Work out the finished part from the listing and answer in its coordinate system (mm). Give positions to 0.01 mm unless a question says otherwise; leave off trailing zeros. Order: outer loops, then holes, each group sorted by start corner. A loop starts at its lowest first (then second) coordinate and runs counter-clockwise, first axis right, second up. Notation, with made-up numbers: (31.25, -28.5) -> (74.25, -28.5) arc R32 cw to (74.25, -0.5) -> close; hole circle Ø5 at (-31, 1). An arc over 180 degrees is marked (long way). Answer as CSV lines item,"result". Start each with the question number.
1. A cutting plane is placed at A-A (z = 1147.5). Give the vertices of the cut face in (x, y), then the cut area to 3 significant figures.
2. A cutting plane is placed at C-C (y = 27). Give the vertices of the cut face in (x, z), then the cut area to 3 significant figures.
3. A cutting plane is placed at B-B (x = 15.5). Give the vertices of the cut face in (y, z).
4. Flat-ended cylindrical pins translate along their axes: pin 1 (3 mm diameter, centred on x = 6.5, y = 11, fed in from +Z); pin 2 (1.5 mm diameter, centred on y = 28, z = 1236.5, fed in from +X); pin 3 (8 mm diameter, centred on x = 25, z = 731, fed in from +Y). Find the tip coordinate at first contact, or state that the pin passes through.
5. Find the intervals of material crossed by L1, parallel to X at y = 3.5, z = 1756; L2, parallel to X at y = 26, z = 1172, in increasing order.
Autodesk Inventor part; units mm, degrees
ref_plane "Start plane" through (0, 0, 0) normal (0, 0, 1) x (1, 0, 0)
ref_plane "End plane" through (0, 0, 1841.5) normal (0, 0, 1) x (1, 0, 0)
ref_plane "Work Plane4" through (19.05, 0, 0) normal (0, 0.7071, -0.7071) x (1, 0, 0)
ref_plane "Start plane" through (0, 0, 0) normal (0, 0, 1) x (1, 0, 0)
ref_plane "End plane" through (0, 0, 1841.5) normal (0, 0, 1) x (1, 0, 0)
sketch "Sketch" plane through (0, 0, 0) normal (0, 0, 1) x (1, 0, 0)
  line L0 (38.1, 0) -> (0, 0)
  line L1 (0, 0) -> (0, 38.1)
  line L2 (0, 38.1) -> (2.4765, 38.1)
  line L3 (4.7625, 35.814) -> (4.7625, 9.5885)
  line L4 (9.5885, 4.7625) -> (35.814, 4.7625)
  line L5 (38.1, 2.4765) -> (38.1, 0)
  line L6 (0, -11.0414) -> (0, 31.5385) construction
  line L7 (-11.0414, 0) -> (31.5385, 0) construction
  arc A0 (4.7625, 9.5885) -> (9.5885, 4.7625) centre (9.5885, 9.5885) ccw
  arc A1 (4.7625, 35.814) -> (2.4765, 38.1) centre (2.4765, 35.814) ccw
  arc A2 (38.1, 2.4765) -> (35.814, 4.7625) centre (35.814, 2.4765) ccw
  line L8 (0, 48.4964) -> (0, -20.9644) construction
  line L9 (-20.9644, 0) -> (48.4964, 0) construction
  point P0 (4.7625, 38.1)
  point P1 (4.7625, 4.7625)
  point P2 (38.1, 4.7625)
  dimension "d0" = 38.1
  dimension "d1" = 38.1
  dimension "d2" = 4.7625
  dimension "d3" = 4.7625
  dimension "d10" = 0
  dimension "d11" = 0
  dimension "d14" = 4.826
  dimension "d15" = 2.286
extrude "Body" add sketch "Sketch" along normal up to surface (1841.5 mm away) from surface at 0
sketch "Sketch3" plane through (0, 0, 0) normal (0, 0, 1) x (1, 0, 0)
  line L0 (0, 0) -> (10, 0)
ref_plane "Work Plane3" through (0, 0, 0) normal (0, -1, 0) x (1, 0, 0)
sketch "Sketch4" plane through (0, 0, 0) normal (0, -1, 0) x (1, 0, 0)
  line L0 (-2, 0) -> (12, 0)
  line L1 (-2, 1841.5) -> (12, 1841.5)
  dimension "d17" = 1841.5
ref_plane "Work Plane4" through (19.05, 0, 0) normal (0, 0.7071, -0.7071) x (1, 0, 0)
split "Split1" plane through (19.05, 0, 0) removes the side toward (0, 0.7071, -0.7071)
ref_plane "Work Plane5" through (19.05, 0, 1841.5) normal (0, 0.7071, 0.7071) x (1, 0, 0)
split "Split2" plane through (19.05, 0, 1841.5) removes the side toward (0, 0.7071, 0.7071)
equation "\"d0\" = G_H"
equation "\"d1\" = G_H"
equation "\"d2\" = G_T"
equation "\"d3\" = G_T"
equation "\"d14\" = G_IR"
equation "\"d15\" = G_ER"
equation "\"d4\" = G_L"
equation "\"G_H\" = 38.1"
equation "\"G_T\" = 4.7625"
equation "\"G_ER\" = 2.286"
equation "\"G_IR\" = 4.826"
equation "\"G_L\" = d17"
equation "\"ex\" = 0"
equation "\"G_OFFSET_START\" = 0"
equation "\"G_OFFSET_END\" = 0"
equation "\"d13\" = G_OFFSET_END + B_L"
equation "\"B_L\" = 1841.5"
properties part number "AISC - L 1.5 x 1.5 x 3/16 - 72.5" material "Aluminum 6061-AHC"
Answer sheet:
1,outline,"(0, 0) -> (38.1, 0) -> (38.1, 2.48) arc R2.29 ccw to (35.81, 4.76) -> (9.59, 4.76) arc R4.83 cw to (4.76, 9.59) -> (4.76, 35.81) arc R2.29 ccw to (2.48, 38.1) -> (0, 38.1) -> close"
1,area,"343 mm^2"
2,outline,"(0, 27) -> (4.76, 27) -> (4.76, 1814.5) -> (0, 1814.5) -> close"
2,area,"8,510 mm^2"
3,outline,"(0, 0) -> (4.76, 4.76) -> (4.76, 1836.74) -> (0, 1841.5) -> close"
4,pin 1,"passes through"
4,pin 2,"stops at x = 4.76"
4,pin 3,"stops at y = 4.76"
5,L1,"x = 0 to 37.86"
5,L2,"x = 0 to 4.76"
